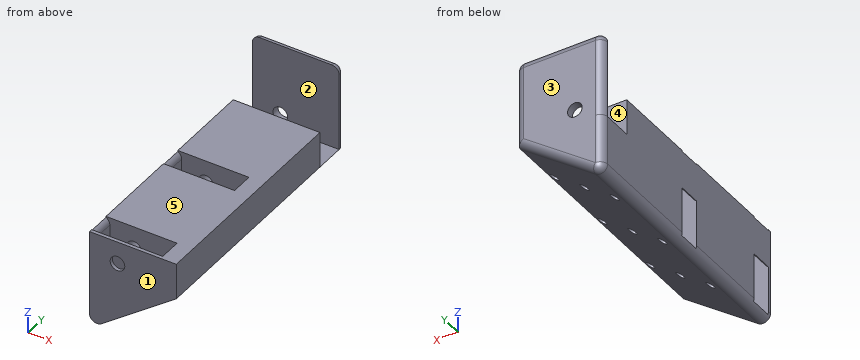
```python
from build123d import *

# Parameters (mm, degrees)
SKETCH1_W               = 29.532117275
SKETCH1_H               = 16.294493356
BOSS_EXTRUDE1_DEPTH     = 6.35
BOSS_EXTRUDE2_DEPTH     = 82.55
SKETCH2_W               = 29.532117275
SKETCH2_H               = 16.294493356
CUT_EXTRUDE1_DEPTH      = 3.175
SKETCH4_W               = 29.532117275
SKETCH4_H               = 12.7
BOSS_EXTRUDE3_DEPTH     = 3.175
SKETCH7_W               = 36.710026843
SKETCH7_H               = 7.62
CUT_EXTRUDE4_DEPTH      = 13.589
SKETCH8_W               = 36.710026843
SKETCH8_H               = 7.62
CUT_EXTRUDE5_DEPTH      = 13.589
SKETCH9_W               = 29.532117275
SKETCH9_H               = 76.2
SKETCH9_W_2             = 22.877365929
SKETCH9_H_2             = 7.62
BOSS_EXTRUDE5_DEPTH     = 12.2428
CUT_EXTRUDE6_DEPTH      = 95.918198917
CUT_EXTRUDE6_DEPTH_BACK = 95.918198917
SKETCH10_R              = 2.4892
FILLET2_R               = 2.54
FILLET3_R               = 2.54
CUT_EXTRUDE7_DEPTH      = 2.54
CUT_EXTRUDE7_DEPTH_BACK = 6.35
SKETCH11_R              = 1.5875
CUT_EXTRUDE8_DEPTH      = 93.343538462
CUT_EXTRUDE8_DEPTH_BACK = 93.343538462
SKETCH12_W              = 28.994493356
SKETCH12_H              = 0.635


with BuildPart() as part:
    # Sketch1 → Boss-Extrude1 (new body)
    with BuildSketch(Plane(origin=(0, 0, 0), x_dir=(1, 0, 0), z_dir=(0, 1, 0))):
        Polygon((16.296436439, 0), (-13.235680836, 21.805506644), (-13.235680836, 0), align=None)
        with Locations((1.530377802, -8.147246678)):
            Rectangle(SKETCH1_W, SKETCH1_H)
    extrude(amount=BOSS_EXTRUDE1_DEPTH)

    # Sketch1<3> → Boss-Extrude2 (add)
    with BuildSketch(Plane(origin=(0, 0, 0), x_dir=(1, 0, 0), z_dir=(0, 1, 0))):
        Polygon((16.296436439, 0), (-13.235680836, 21.805506644), (-13.235680836, 0), align=None)
    extrude(amount=-BOSS_EXTRUDE2_DEPTH)

    # Sketch2 → Cut-Extrude1 (cut)
    with BuildSketch(Plane(origin=(0, 0, 0), x_dir=(-1, 0, 0), z_dir=(0, -1, 0))):
        with Locations((-1.530377802, -8.147246678)):
            Rectangle(SKETCH2_W, SKETCH2_H)
    extrude(amount=-CUT_EXTRUDE1_DEPTH, mode=Mode.SUBTRACT)

    # Sketch4 → Boss-Extrude3 (add)
    with BuildSketch(Plane(origin=(0, 6.35, 0), x_dir=(1, 0, 0), z_dir=(0, 1, 0))):
        with Locations((1.530377802, -22.644493356)):
            Rectangle(SKETCH4_W, SKETCH4_H)
    extrude(amount=-BOSS_EXTRUDE3_DEPTH)

    # Sketch7 → Cut-Extrude4 (cut)
    with BuildSketch(Plane(origin=(3.863909533, 0, -5.233055638), x_dir=(-0.804470053980136, 0, -0.5939932089251503), z_dir=(0.5939932089251503, 0, -0.804470053980136))):
        with Locations((5.24501832, -77.597)):
            Rectangle(SKETCH7_W, SKETCH7_H)
    extrude(amount=-CUT_EXTRUDE4_DEPTH, mode=Mode.SUBTRACT)

    # Sketch8 → Cut-Extrude5 (cut)
    with BuildSketch(Plane(origin=(3.863909533, 0, -5.233055638), x_dir=(-0.804470053980136, 0, -0.5939932089251503), z_dir=(0.5939932089251503, 0, -0.804470053980136))):
        with Locations((5.24501832, -39.497)):
            Rectangle(SKETCH8_W, SKETCH8_H)
    extrude(amount=-CUT_EXTRUDE5_DEPTH, mode=Mode.SUBTRACT)

    # Sketch9 → Boss-Extrude5 (add)
    with BuildSketch(Plane.XY):
        with Locations((1.530377802, -44.45)):
            Rectangle(SKETCH9_W, SKETCH9_H)
        with Locations((-0.487425481, -77.597)):
            Rectangle(SKETCH9_W_2, SKETCH9_H_2, mode=Mode.SUBTRACT)
        with Locations((-0.487425481, -39.497)):
            Rectangle(SKETCH9_W_2, SKETCH9_H_2, mode=Mode.SUBTRACT)
    extrude(amount=BOSS_EXTRUDE5_DEPTH)

    # Sketch10 → Cut-Extrude6 (cut, two sides: drawn at the far end of the back side and taken through both)
    with BuildSketch(Plane(origin=(0, -82.55, 0), x_dir=(-1, 0, 0), z_dir=(0, -1, 0)).offset(-CUT_EXTRUDE6_DEPTH_BACK)):
        with Locations(Location((3.710680836, -4.6228, 0), (0, 0, 270))):
            Circle(SKETCH10_R)
    extrude(amount=CUT_EXTRUDE6_DEPTH + CUT_EXTRUDE6_DEPTH_BACK, mode=Mode.SUBTRACT)

    # Fillet2
    # the kernel refuses this fillet: 2.54 mm, written as the material it takes off along each edge
    with BuildSketch(Plane(origin=(-13.235680836, -95.13201822, -21.805506644), x_dir=(0.8044700539801357, 0, 0.5939932089251506), z_dir=(0, 1, 0))) as fillet2_piece_1:
        with BuildLine():
            CenterArc((FILLET2_R * 1.98142019214, -FILLET2_R), FILLET2_R, 90, 126.440893479)
            Line((FILLET2_R * 1.17695013816, -FILLET2_R * 1.59399320893), (0, 0))
            Line((0, 0), (FILLET2_R * 1.98142019214, 0))
        make_face()
    extrude(amount=114.06403644, mode=Mode.SUBTRACT)
    with BuildSketch(Plane(origin=(-11.926108446, -81.407, 0), x_dir=(-0.8044700539801358, 0, -0.5939932089251506), z_dir=(0, 1, 0))) as fillet2_piece_2:
        with BuildLine():
            CenterArc((FILLET2_R * 0.504688507753, FILLET2_R), FILLET2_R, 216.440893479, 53.559106521)
            Line((-FILLET2_R * 0.299781546228, FILLET2_R * 0.406006791075), (0, 0))
            Line((0, 0), (FILLET2_R * 0.504688507753, 0))
        make_face()
    extrude(amount=7.62, mode=Mode.SUBTRACT)
    with BuildSketch(Plane(origin=(-11.926108446, -81.407, 12.2428), x_dir=(-1, 0, 0), z_dir=(0, 1, 0)), Plane(origin=(-11.926108446, -43.307, 12.2428), x_dir=(-1, 0, 0), z_dir=(0, 1, 0))) as fillet2_piece_3:
        with BuildLine():
            CenterArc((FILLET2_R, -FILLET2_R), FILLET2_R, 90, 90)
            Line((0, -FILLET2_R), (0, 0))
            Line((0, 0), (FILLET2_R, 0))
        make_face()
    extrude(amount=7.62, mode=Mode.SUBTRACT)
    with BuildSketch(Plane(origin=(-11.926108446, -35.687, 0), x_dir=(-0.8044700539801356, 0, -0.5939932089251507), z_dir=(0, -1, 0))) as fillet2_piece_4:
        with BuildLine():
            CenterArc((FILLET2_R * 0.504688507753, -FILLET2_R), FILLET2_R, 90, 53.559106521)
            Line((-FILLET2_R * 0.299781546228, -FILLET2_R * 0.406006791075), (0, 0))
            Line((0, 0), (FILLET2_R * 0.504688507753, 0))
        make_face()
    extrude(amount=7.62, mode=Mode.SUBTRACT)
    with BuildSketch(Plane(origin=(-13.235680836, 12.7, 28.994493356), x_dir=(0, 0, -1), z_dir=(0, -1, 0))) as fillet2_piece_5:
        with BuildLine():
            CenterArc((FILLET2_R, FILLET2_R), FILLET2_R, 180, 90)
            Line((0, FILLET2_R), (0, 0))
            Line((0, 0), (FILLET2_R, 0))
        make_face()
    extrude(amount=15.875, mode=Mode.SUBTRACT)
    with BuildSketch(Plane(origin=(16.296436439, 12.7, 28.994493356), x_dir=(0, 0, -1), z_dir=(0, -1, 0))) as fillet2_piece_6:
        with BuildLine():
            CenterArc((FILLET2_R, -FILLET2_R), FILLET2_R, 90, 90)
            Line((0, -FILLET2_R), (0, 0))
            Line((0, 0), (FILLET2_R, 0))
        make_face()
    extrude(amount=15.875, mode=Mode.SUBTRACT)

    # Fillet3
    fillet3_edges = [part.edges().sort_by_distance(p)[0] for p in [
        (-13.235680836, 6.35, 4.840897),
        (1.530377801, 6.35, 28.994493356),
        (16.296436439, 6.35, 13.227246678),
        (15.552487663, 6.35, 28.25054458),
        (-12.491732061, 6.35, 28.25054458),
        (-11.840100649, 6.35, -19.04027588),
        (3.554749177, 6.35, -9.408026646),
    ]]
    fillet(fillet3_edges, radius=FILLET3_R)

    # Sketch11 → Cut-Extrude7 (cut, two sides: drawn at the far end of the back side and taken through both)
    with BuildSketch(Plane(origin=(5.749837972, 0, -7.787248059), x_dir=(-0.8044700539801359, 0, -0.5939932089251502), z_dir=(0.5939932089251502, 0, -0.8044700539801359)).offset(-CUT_EXTRUDE7_DEPTH_BACK)):
        with Locations(Location((-11.04569204, -62.23, 0), (0, 0, 180))):
            Circle(SKETCH11_R)
        with Locations(Location((1.65430796, -62.23, 0), (0, 0, 180))):
            Circle(SKETCH11_R)
        with Locations(Location((14.35430796, -62.23, 0), (0, 0, 180))):
            Circle(SKETCH11_R)
        with Locations(Location((-11.04569204, -36.83, 0), (0, 0, 180))):
            Circle(SKETCH11_R)
        with Locations(Location((1.65430796, -36.83, 0), (0, 0, 180))):
            Circle(SKETCH11_R)
        with Locations(Location((14.35430796, -36.83, 0), (0, 0, 180))):
            Circle(SKETCH11_R)
        with Locations(Location((-11.04569204, -11.43, 0), (0, 0, 180))):
            Circle(SKETCH11_R)
        with Locations(Location((1.65430796, -11.43, 0), (0, 0, 180))):
            Circle(SKETCH11_R)
        with Locations(Location((14.35430796, -11.43, 0), (0, 0, 180))):
            Circle(SKETCH11_R)
    extrude(amount=CUT_EXTRUDE7_DEPTH + CUT_EXTRUDE7_DEPTH_BACK, mode=Mode.SUBTRACT)

    # Sketch12 → Cut-Extrude8 (cut, two sides: drawn at the far end of the back side and taken through both)
    with BuildSketch(Plane(origin=(16.296436439, 0, 0), x_dir=(0, 0, -1), z_dir=(1, 0, 0)).offset(-CUT_EXTRUDE8_DEPTH_BACK)):
        with Locations((-14.497246678, 3.4925)):
            Rectangle(SKETCH12_W, SKETCH12_H)
    extrude(amount=CUT_EXTRUDE8_DEPTH + CUT_EXTRUDE8_DEPTH_BACK, mode=Mode.SUBTRACT)


solid = part.part
```
Source: CAD feature listing. Evaluate the final solid. Frame: model axes, mm. Face numbers are marked on the shaded views. A direction names the side the tool comes from. Round coordinates to 2 decimals unless told otherwise and drop trailing zeros. Loops run counter-clockwise (first coordinate to the right, second up) from the corner with the lowest first, then second, coordinate; pieces in that order, holes last.
1. Section query A-A on z = 8.5. Output: boundary loops of the cut face in (x, y).
2. Section query D-D on z = 19. Output: boundary loops of the cut face in (x, y).
3. Contact query for flat-ended pins moving along their axis: pin 1 (3 mm diameter, centred on x = -10, y = -31, fed in from +Z); pin 2 (3 mm diameter, centred on x = -3.71, z = 4.62, fed in from -Y); pin 3 (4 mm diameter, centred on x = 2, z = 15.5, fed in from -Y). Output: stop coordinate, or through.
4. Section query C-C on y = -58. Output: boundary loops of the cut face in (x, z).
5. Access query for the marked faces 1 and 2. Directions: +Z, -Z, +X, -X, +Y, -Y. A direction counts if a zero-diameter tool reaches every point of the face in a straight line with its end or side. Return the directions, or none.
6. Section query B-B on y = -40. Output: boundary loops of the cut face in (x, z), and give its area (3 significant figures).
7. Mould query, pull axis Y, two halves, no side actions, for the marked faces 3, 4 and 5. Classes: released by +Y, released by -Y, zero draft, split by the parting line, or undercut.
8. Ray query, L1, parallel to Y at x = -9, z = -8; L2, parallel to Y at x = 0.75, z = 3. Return the intervals inside material, ascending.
Answers below:
1. outline: (-13.24, -82.55) - (16.3, -82.55) - (16.3, -6.35) - (-13.24, -6.35) - close; (-13.24, 3.81) - (16.3, 3.81) arc R2.54 ccw to (13.76, 6.35) - (-10.7, 6.35) arc R2.54 ccw to start; hole (-11.93, -81.41) - (10.95, -81.41) - (10.95, -73.79) - (-11.93, -73.79) - close; hole (-11.93, -43.31) - (10.95, -43.31) - (10.95, -35.69) - (-11.93, -35.69) - close
2. outline: (-13.24, 3.81) - (16.3, 3.81) arc R2.54 ccw to (13.76, 6.35) - (-10.7, 6.35) arc R2.54 ccw to start
3. pin 1: stops at z = 12.24
3. pin 2: passes through
3. pin 3: stops at y = 3.81
4. outline: (-13.24, -16.77) arc R2.54 ccw to (-9.19, -18.82) - (16.3, 0) - (16.3, 12.24) - (-13.24, 12.24) - close; hole circle Ø4.98 at (-3.71, 4.62)
5. face 1: +Z, -Z, +X, -X, -Y
5. face 2: +Z, +X, -X
6. outline: (-13.24, -0.97) - (-12.96, -0.76) arc R2.54 ccw to (-11.93, 1.28) - (-11.93, 9.7) arc R2.54 ccw to (-13.24, 11.92) - close; (-13.05, -17.72) arc R2.54 ccw to (-9.19, -18.82) - (16.3, 0) - (16.3, 12.24) - (10.95, 12.24) - (10.95, 0) - close
6. area: 181 mm2
7. face 3: released by +Y
7. face 4: undercut
7. face 5: zero draft
8. L1: y = -82.55 to -81.41, -73.79 to -43.31, -35.69 to 6.35
8. L2: y = -82.55 to -81.41, -73.79 to -43.31, -35.69 to -6.35, 3.81 to 6.35
